from build123d import *

# Parameters (mm, degrees)
SKETCH1_W           = 100
SKETCH1_H           = 50
BOSS_EXTRUDE1_DEPTH = 3
SKETCH2_W           = 60
SKETCH2_H           = 15
CUT_EXTRUDE1_DEPTH  = 3
FILLET1_R           = 7.4
SKETCH3_W           = 3
SKETCH3_H           = 20
SKETCH3_H_2         = 10
CUT_EXTRUDE2_DEPTH  = 10
SKETCH4_W           = 10
SKETCH4_H           = 3
CUT_EXTRUDE3_DEPTH  = 3


with BuildPart() as part:
    # Sketch1 → Boss-Extrude1 (new body)
    with BuildSketch(Plane(origin=(0, 0, 0), x_dir=(1, 0, 0), z_dir=(0, 1, 0))):
        with Locations((50, 25)):
            Rectangle(SKETCH1_W, SKETCH1_H)
    extrude(amount=BOSS_EXTRUDE1_DEPTH)

    # Sketch2 → Cut-Extrude1 (cut)
    with BuildSketch(Plane(origin=(0, 3, 0), x_dir=(1, 0, 0), z_dir=(0, 1, 0))):
        with Locations((70, 7.5)):
            Rectangle(SKETCH2_W, SKETCH2_H)
        with Locations((70, 42.5)):
            Rectangle(SKETCH2_W, SKETCH2_H)
    extrude(amount=-CUT_EXTRUDE1_DEPTH, mode=Mode.SUBTRACT)

    # Fillet1
    fillet1_edges = [part.edges().sort_by_distance(p)[0] for p in [
        (100, 1.5, -15),
        (40, 1.5, 0),
        (40, 1.5, -15),
        (100, 1.5, -35),
        (40, 1.5, -35),
        (40, 1.5, -50),
        (0, 1.5, -50),
        (0, 1.5, 0),
    ]]
    fillet(fillet1_edges, radius=FILLET1_R)

    # Sketch3 → Cut-Extrude2 (cut)
    with BuildSketch(Plane.XZ):
        with Locations((21.5, -25)):
            Rectangle(SKETCH3_W, SKETCH3_H)
        with Locations((78.5, -25)):
            Rectangle(SKETCH3_W, SKETCH3_H_2)
    extrude(amount=-CUT_EXTRUDE2_DEPTH, mode=Mode.SUBTRACT)

    # Sketch4 → Cut-Extrude3 (cut)
    with BuildSketch(Plane.XZ):
        with Locations((30.91970706, -19.5)):
            Rectangle(SKETCH4_W, SKETCH4_H)
        with Locations((65.91970706, -19.5)):
            Rectangle(SKETCH4_W, SKETCH4_H)
    extrude(amount=-CUT_EXTRUDE3_DEPTH, mode=Mode.SUBTRACT)


solid = part.part
Check sheet for the modelled part. Datum: model origin and axes. Units: mm. A direction names the side the tool comes from. Round coordinates to 2 decimals unless told otherwise and drop trailing zeros. Loops run counter-clockwise (first coordinate to the right, second up) from the corner with the lowest first, then second, coordinate; pieces in that order, holes last. Notation, with made-up numbers: (45.5, 73.5) -> (98.5, 73.5) arc R31 ccw to (98.5, 110.5) -> close; hole circle Ø7 at (26.25, 61). An arc over 180 degrees is marked (long way). Put each result on its own line as item: value. Start each with the question number.
1. Section check B-B (y = 1.6). Give the number of separate pieces and of enclosed holes in the cut face, plus the area to 3 significant figures.
2. Draft check along Z on faces 4 (the face through (35.92, 1, -20)), 5 (the face through (20, 1, 0)), 6 (the face through (77, 1, -25)), 7 (the face through (38, 0, -25)). Enter one of: +Z half, -Z half, draft (parallel to the pull), parting line (faces both ways), or undercut.
3. Access from +Z, -Z, +X, -X, +Y, -Y to the whole of each face (thin tool, end or side, straight path). Record for faces 1 (the face through (70, 2, -15)), 2 (the face through (2.11, 1.521, -2.225)), 3 (the face through (31, 1, -18)).
4. Gauge pin test, flat ends, axial feed: pin 1 (1.5 mm diameter, centred on x = 79, y = 1, fed in from +Z); pin 2 (1.5 mm diameter, centred on x = 78, y = 1, fed in from -Z); pin 3 (10 mm diameter, centred on x = 47, z = -21, fed in from -Y); pin 4 (1 mm diameter, centred on y = 1, z = -19.5, fed in from +X). Record the tip position at first contact, or that the pin passes through.
5. Scan lines: probe 1 along X at (y, z) = (0.55, -24); probe 2 along X at (y, z) = (0.2, -19); probe 3 along Z at (x, y) = (26.5, 1.3). Record each from-to range of solid material in increasing order.
6. Section check A-A (x = 31). Enter the section's corners in (y, z), plus the area to 3 significant figures.
7. Section check D-D (x = 91.5). Enter the section's corners in (y, z).
8. Section check C-C (z = -33). Enter the section's corners in (x, y).
Findings:
1. separate pieces: 1
1. enclosed holes: 4
1. area: 3,000 mm^2
2. face 4: undercut
2. face 5: +Z half
2. face 6: undercut
2. face 7: draft
3. face 1: +Z, +X, +Y, -Y
3. face 2: +Z, -X, +Y, -Y
3. face 3: +Y, -Y
4. pin 1: stops at z = -15
4. pin 2: stops at z = -35
4. pin 3: stops at y = 0
4. pin 4: stops at x = 99.6
5. probe 1: x = 0 to 20, 23 to 77, 80 to 100
5. probe 2: x = 0 to 20, 23 to 25.92, 35.92 to 60.92, 70.92 to 99.17
5. probe 3: z = -50 to -21, -18 to 0
6. outline: (0, -50) -> (3, -50) -> (3, -21) -> (0, -21) -> close; (0, -18) -> (3, -18) -> (3, 0) -> (0, 0) -> close
6. area: 141 mm^2
7. outline: (0, -35) -> (3, -35) -> (3, -15) -> (0, -15) -> close
8. outline: (0, 0) -> (20, 0) -> (20, 3) -> (0, 3) -> close; (23, 0) -> (97.66, 0) -> (97.66, 3) -> (23, 3) -> close
